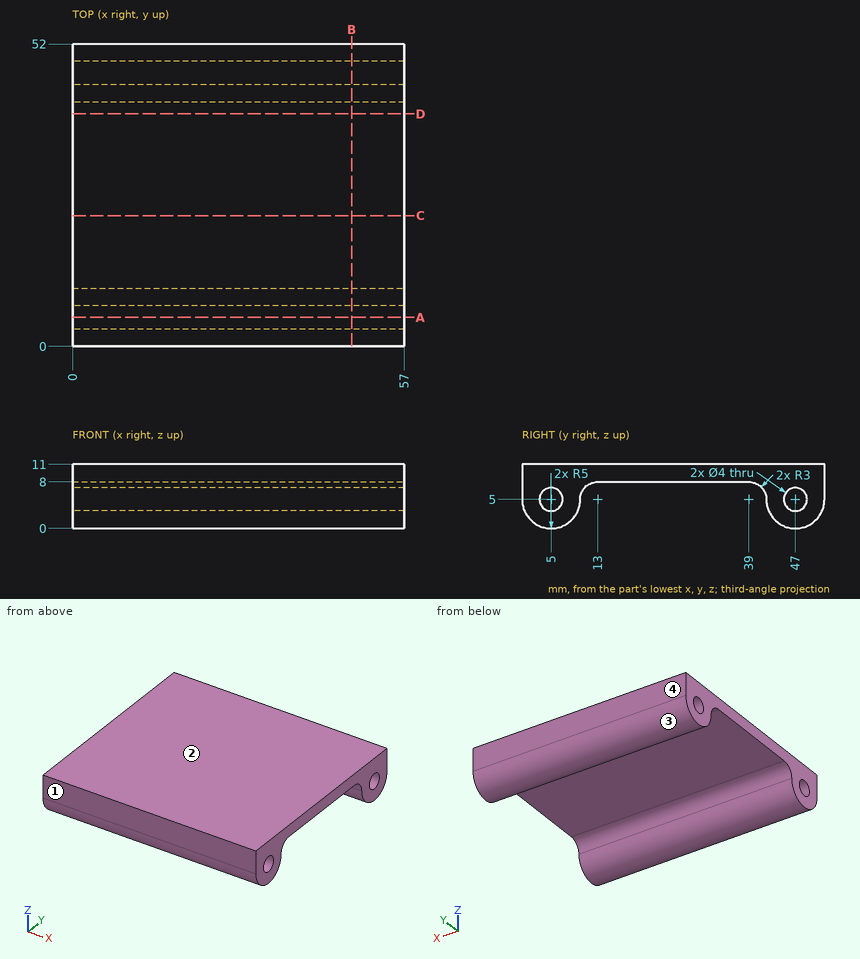
Can you work these out from the drawing? Everything is in mm from the part's minimum corner. Round coordinates to 2 decimals unless told otherwise and drop trailing zeros. Loops run counter-clockwise (first coordinate to the right, second up) from the corner with the lowest first, then second, coordinate; pieces in that order, holes last.
1. If we section it at B-B on x = 48: Write out the boundary of the cut face in (y, z), plus the area to 3 significant figures.
Answer list:
outline: (0, 5) arc R5 ccw to (10, 5) arc R3 cw to (13, 8) - (39, 8) arc R3 cw to (42, 5) arc R5 ccw to (52, 5) - (52, 11) - (0, 11) - close; hole circle Ø4 at (5, 5); hole circle Ø4 at (47, 5)
area: 273 mm2
2. If we section it at A-A on y = 5: Write out the boundary of the cut face in (x, z).
Answer list:
outline: (0, 0) - (57, 0) - (57, 3) - (0, 3) - close; (0, 7) - (57, 7) - (57, 11) - (0, 11) - close
3. If I drill on line 1 along Y through (x, z) = (37.5, 5); line 2 along Z through (x, y) = (42, 47); line 3 along Z through (x, y) = (8, 14), over which ranges is the centre line in solid material (lowest first)?
Answer list:
line 1: y = 0 to 3, 7 to 10, 42 to 45, 49 to 52
line 2: z = 0 to 3, 7 to 11
line 3: z = 8 to 11
4. We'd pull the mould along Y, two halves only. Please class the marked faces 1, 2, 3 and 4: +Y half, -Y half, draft (parallel to the pull), parting line (faces both ways), or undercut.
Answer list:
face 1: -Y half
face 2: draft
face 3: undercut
face 4: +Y half
5. For P1, Ø1.5, axis at x = 25, y = 13.5, coming from the -Z side, with a flat end and sliding along its axis, tell me the tip position at first contact or that it passes through.
Answer list:
P1: stops at z = 7.99
6. If we section it at D-D on y = 40: Write out the boundary of the cut face in (x, z), plus the area to 3 significant figures.
Answer list:
outline: (0, 7.83) - (57, 7.83) - (57, 11) - (0, 11) - close
area: 181 mm2
7. If we section it at C-C on y = 22.5: Write out the boundary of the cut face in (x, z).
Answer list:
outline: (0, 8) - (57, 8) - (57, 11) - (0, 11) - close
